from build123d import *

# Parameters (mm, degrees)
SKETCH_1_R          = 11.5
EXTRUDE_1_DEPTH     = 16
EXTRUDE_START       = -3
SKETCH_2_R          = 12.5
EXTRUDE_2_DEPTH     = 4
SKETCH_3_R          = 9.75
CUT_EXTRUDE_1_DEPTH = 2
SKETCH_4_R          = 9
CUT_EXTRUDE_2_DEPTH = 23.549944568
SKETCH_5_R          = 10
CUT_EXTRUDE_3_DEPTH = 11
CHAMFER_1_SIZE      = 0.5
FILLET_1_R          = 0.5


with BuildPart() as part:
    # 草图1 → 凸台-拉伸1 (new body)
    with BuildSketch(Plane.XY):
        Circle(SKETCH_1_R)
    extrude(amount=EXTRUDE_1_DEPTH)

    # 草图2 → 凸台-拉伸2 (add)
    with BuildSketch(Plane.XY.offset(16).offset(EXTRUDE_START)):
        Circle(SKETCH_2_R)
    extrude(amount=-EXTRUDE_2_DEPTH)

    # 草图3 → 切除-拉伸1 (cut)
    with BuildSketch(Plane.XY.offset(16)):
        Circle(SKETCH_3_R)
    extrude(amount=-CUT_EXTRUDE_1_DEPTH, mode=Mode.SUBTRACT)

    # 草图4 → 切除-拉伸2 (cut, through all)
    with BuildSketch(Plane.XY.offset(14)):
        Circle(SKETCH_4_R)
    extrude(amount=-CUT_EXTRUDE_2_DEPTH, mode=Mode.SUBTRACT)

    # 草图5 → 切除-拉伸3 (cut)
    with BuildSketch(Plane(origin=(0, 0, 0), x_dir=(-1, 0, 0), z_dir=(0, 0, -1))):
        Circle(SKETCH_5_R)
    extrude(amount=-CUT_EXTRUDE_3_DEPTH, mode=Mode.SUBTRACT)

    # 倒角1
    chamfer_1_edges = [part.edges().sort_by_distance(p)[0] for p in [
        (-9.75, 0, 16),
        (-9, 0, 14),
        (10, 0, 0),
        (-11.5, 0, 16),
    ]]
    chamfer(chamfer_1_edges, length=CHAMFER_1_SIZE)

    # 圆角1
    fillet_1_edges = [part.edges().sort_by_distance(p)[0] for p in [
        (-12.5, 0, 9),
        (-12.5, 0, 13),
    ]]
    fillet(fillet_1_edges, radius=FILLET_1_R)


solid = part.part
Model file for the job. Use its own axes, mm. A direction names the side the tool comes from. Coordinates: 2 decimals unless noted, no trailing zeros. Write each loop counter-clockwise with the first axis right and the second up, starting at its lowest first coordinate (ties: lowest second). Pieces come first, ordered by that corner, then holes. Notation, with made-up numbers: (89.25, 36) - (129.25, 36) arc R25 cw to (129.25, 51) - close; hole circle Ø5 at (74.5, 65). An arc over 180 degrees is marked (long way). Write each question's results on one line, items separated by ' | '. Start each with the question number.
1) Flat gauge pins, fed straight in: P1, Ø3, axis at y = 8.5, z = 13, coming from the -X side; P2, Ø5, axis at y = 3, z = 2.5, coming from the +X side; P3, Ø1, axis at x = -5, z = 7.5, coming from the +Y side; P4, Ø7, axis at x = -5, y = -2, coming from the +Z side. Where does each tip first touch, or does it go through?
2) Cut at B-B (z = 10.25). Write the cut outline in (x, y), then the cut area to 3 significant figures.
3) Cut at A-A (z = 7.5). Write the cut outline in (x, y), then the cut area to 3 significant figures.
4) Mould opens along Y. For faces 1 (the face through (3.4, -10.2, 0)), 2 (the face through (-1.5, 11.4, 4.4)), 3 (the face through (-1.269, 9.667, 14.76)) say: pulls with the +Y half, pulls with the -Y half, needs draft (parallel to the pull), parting line crosses it, or undercut.
5) Probe line 1 along Y through (x, z) = (0, 12); line 2 along Z through (x, y) = (5.75, 10); line 3 along Y through (x, z) = (-4.75, 1.75). List the from-to ranges inside material, lowest first. Write a range as from..to.
6) 3-axis set-ups, long thin cutter, end or side, ignore diameter. For faces 4 (the face through (-1.5, 11.4, 14.2)), 5 (the face through (-1.172, 8.923, 12.268)), 6 (the face through (9, 2, 11)): which of +Z, -Z, +X, -X, +Y, -Y reach the whole face in a straight line?
Returned:
1) P1: x = -10.31 | P2: x = 11.49 | P3: y = 10.58 | P4: through
2) outline: circle Ø25 at (0, 0); hole circle Ø20 at (0, 0) | area: 177 mm^2
3) outline: circle Ø23 at (0, 0); hole circle Ø20 at (0, 0) | area: 101 mm^2
4) face 1: needs draft | face 2: parting line crosses it | face 3: undercut
5) line 1: -12.5..-9, 9..12.5 | line 2: 9..13 | line 3: -10.47..-8.8, 8.8..10.47
6) face 4: +Z | face 5: +Z, -Z | face 6: -Z
